from build123d import *

# Parameters (mm, degrees)
SKETCH1_R           = 6.339
SKETCH1_R_2         = 3.302
SKETCH1_R_3         = 11
BOSS_EXTRUDE1_DEPTH = 3.175


with BuildPart() as part:
    # Sketch1 → Boss-Extrude1 (new body)
    with BuildSketch(Plane(origin=(0, 0, 0), x_dir=(1, 0, 0), z_dir=(0, 1, 0))):
        with BuildLine():
            ThreePointArc((-17.674506033, 5.017864634), (-12.991672891, 12.991672891), (-5.017864634, 17.674506033))
            ThreePointArc((-5.017864634, 17.674506033), (-5.832389069, 19.064824865), (-6.270051206, 20.615595113))
            ThreePointArc((-6.270051206, 20.615595113), (-15.236736921, 15.236736921), (-20.615595113, 6.270051206))
            ThreePointArc((-20.615595113, 6.270051206), (-19.064824865, 5.832389069), (-17.674506033, 5.017864634))
        make_face()
        with Locations((-21.548, 0)):
            Circle(SKETCH1_R)
        with Locations((-21.548, 0)):
            Circle(SKETCH1_R_2, mode=Mode.SUBTRACT)
        with BuildLine():
            ThreePointArc((-17.674506033, -5.017864634), (-19.064824865, -5.832389069), (-20.615595113, -6.270051206))
            ThreePointArc((-20.615595113, -6.270051206), (-15.236736921, -15.236736921), (-6.270051206, -20.615595113))
            ThreePointArc((-6.270051206, -20.615595113), (-5.832389069, -19.064824865), (-5.017864634, -17.674506033))
            ThreePointArc((-5.017864634, -17.674506033), (-12.991672891, -12.991672891), (-17.674506033, -5.017864634))
        make_face()
        with Locations((0, -21.548)):
            Circle(SKETCH1_R)
        with Locations((0, -21.548)):
            Circle(SKETCH1_R_2, mode=Mode.SUBTRACT)
        with BuildLine():
            ThreePointArc((-9.788821916, -5.017864634), (-10.999995425, -0.010032833), (-9.797958971, 5))
            Line((-9.797958971, 5), (-17.651473213, 5))
            ThreePointArc((-17.651473213, 5), (-15.852255786, 2.782340534), (-15.209, 0))
            ThreePointArc((-15.209, 0), (-15.85866791, -2.795428656), (-17.674506033, -5.017864634))
            Line((-17.674506033, -5.017864634), (-9.788821916, -5.017864634))
        make_face()
        with BuildLine():
            ThreePointArc((5.017864634, -9.788821916), (0.010032833, -10.999995425), (-5, -9.797958971))
            Line((-5, -9.797958971), (-5, -17.651473213))
            ThreePointArc((-5, -17.651473213), (0.014574429, -15.209016755), (5.017864634, -17.674506033))
            Line((5.017864634, -17.674506033), (5.017864634, -9.788821916))
        make_face()
        Circle(SKETCH1_R_3)
        Polygon((5, 2.886751346), (0, 5.773502692), (-5, 2.886751346), (-5, -2.886751346), (0, -5.773502692), (5, -2.886751346), align=None, mode=Mode.SUBTRACT)
        with BuildLine():
            ThreePointArc((5, 17.651473213), (-0.014574429, 15.209016755), (-5.017864634, 17.674506033))
            Line((-5.017864634, 17.674506033), (-5.017864634, 9.788821916))
            ThreePointArc((-5.017864634, 9.788821916), (-0.010032833, 10.999995425), (5, 9.797958971))
            Line((5, 9.797958971), (5, 17.651473213))
        make_face()
        with Locations((0, 21.548)):
            Circle(SKETCH1_R)
        with Locations((0, 21.548)):
            Circle(SKETCH1_R_2, mode=Mode.SUBTRACT)
        with BuildLine():
            ThreePointArc((6.270051206, 20.615595113), (5.832389069, 19.064824865), (5.017864634, 17.674506033))
            ThreePointArc((5.017864634, 17.674506033), (12.991672891, 12.991672891), (17.674506033, 5.017864634))
            ThreePointArc((17.674506033, 5.017864634), (19.064824865, 5.832389069), (20.615595113, 6.270051206))
            ThreePointArc((20.615595113, 6.270051206), (15.236736921, 15.236736921), (6.270051206, 20.615595113))
        make_face()
        with BuildLine():
            Line((17.674506033, 5.017864634), (9.788821916, 5.017864634))
            ThreePointArc((9.788821916, 5.017864634), (10.692919178, 2.580984204), (11, 0))
            ThreePointArc((11, 0), (10.695268783, -2.571230378), (9.797958971, -5))
            Line((9.797958971, -5), (17.651473213, -5))
            ThreePointArc((17.651473213, -5), (15.209016755, 0.014574429), (17.674506033, 5.017864634))
        make_face()
        with Locations((21.548, 0)):
            Circle(SKETCH1_R)
        with Locations((21.548, 0)):
            Circle(SKETCH1_R_2, mode=Mode.SUBTRACT)
        with BuildLine():
            ThreePointArc((20.615595113, -6.270051206), (19.064824865, -5.832389069), (17.674506033, -5.017864634))
            ThreePointArc((17.674506033, -5.017864634), (12.991672891, -12.991672891), (5.017864634, -17.674506033))
            ThreePointArc((5.017864634, -17.674506033), (5.832389069, -19.064824865), (6.270051206, -20.615595113))
            ThreePointArc((6.270051206, -20.615595113), (15.236736921, -15.236736921), (20.615595113, -6.270051206))
        make_face()
    extrude(amount=BOSS_EXTRUDE1_DEPTH)


solid = part.part
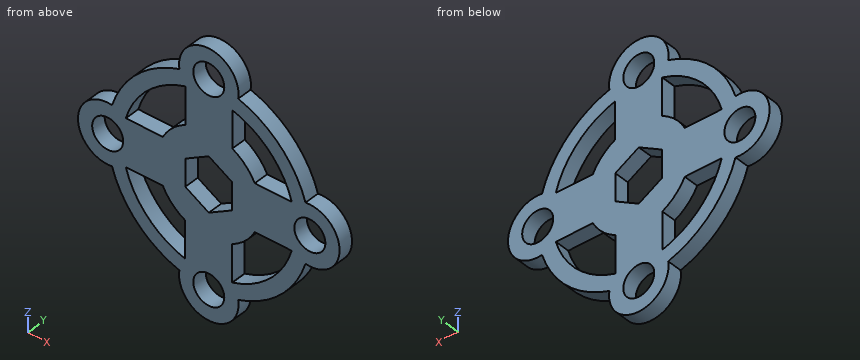
Design review of the part built by this model. Coordinates are the model's own, in mm. Give positions to 0.01 mm unless a question says otherwise; leave off trailing zeros. Order: outer loops, then holes, each group sorted by start corner. A loop starts at its lowest first (then second) coordinate and runs counter-clockwise, first axis right, second up.
1. For pin 1 Ø1.6 at (x, y) = (14.5, 2) entering from -Z; pin 2 Ø1 at (x, y) = (-12, 2) entering from +Z; pin 3 Ø1 at (y, z) = (1.5, 15) entering from -X, all flat-tipped, find the tip position at first contact; note any pin that passes through.
Solution:
pin 1: stops at z = -16.63
pin 2: stops at z = 18.22
pin 3: stops at x = -15.94
2. To check wall thickness, follow L1, parallel to Z at x = 0, y = 1.25; L2, parallel to X at y = 1.15, z = 0; L3, parallel to X at y = 2.1, z = 10. State the ranges of each line that lie inside material, in increasing order.
Solution:
L1: z = -27.89 to -24.85, -18.25 to -5.77, 5.77 to 18.25, 24.85 to 27.89
L2: x = -27.89 to -24.85, -18.25 to -5, 5 to 18.25, 24.85 to 27.89
L3: x = -19.09 to -15.41, -5 to 5.02, 15.41 to 19.09
3. Add section D-D, the plane y = 1.95. State how many separate pieces and enclosed holes the cut face has, then the cut area to 3 significant figures.
Solution:
separate pieces: 1
enclosed holes: 9
area: 1,120 mm2
4. Add section C-C, the plane x = 23.5. State the section outline as (y, z) points (3 decimals), then the cut area to 3 significant figures.
Solution:
outline: (0, -6.031) - (3.175, -6.031) - (3.175, -2.663) - (0, -2.663) - close; (0, 2.663) - (3.175, 2.663) - (3.175, 6.031) - (0, 6.031) - close
area: 21.4 mm2
5. Add section B-B, the plane x = 12.5. State the section outline as (y, z) points (3 decimals), then the cut area to 3 significant figures.
Solution:
outline: (0, -17.552) - (3.175, -17.552) - (3.175, -13.465) - (0, -13.465) - close; (0, -5.018) - (3.175, -5.018) - (3.175, 5) - (0, 5) - close; (0, 13.465) - (3.175, 13.465) - (3.175, 17.552) - (0, 17.552) - close
area: 57.8 mm2
6. Add section A-A, the plane z = 0. State the section outline as (x, y) points (3 decimals), then the cut area to 3 significant figures.
Solution:
outline: (-27.887, 0) - (-24.85, 0) - (-24.85, 3.175) - (-27.887, 3.175) - close; (-18.246, 0) - (-5, 0) - (-5, 3.175) - (-18.246, 3.175) - close; (5, 0) - (18.246, 0) - (18.246, 3.175) - (5, 3.175) - close; (24.85, 0) - (27.887, 0) - (27.887, 3.175) - (24.85, 3.175) - close
area: 103 mm2
